Autodesk Inventor part; units mm, degrees
ref_plane "YZ Plane" through (0, 0, 0) normal (1, 0, 0) x (0, 1, 0)
ref_plane "XZ Plane" through (0, 0, 0) normal (0, 1, 0) x (-1, 0, 0)
ref_plane "XY Plane" through (0, 0, 0) normal (0, 0, 1) x (1, 0, 0)
sketch "Sketch1" plane through (0, 0, 0) normal (0, 0, 1) x (1, 0, 0)
  line L0 (-14, 8) -> (14, 8)
  line L1 (14, 8) -> (14, -8)
  line L2 (14, -8) -> (-14, -8)
  line L3 (-14, -8) -> (-14, 8)
  circle A0 centre (-9, 4) radius 1.6
  circle A1 centre (-9, -4) radius 1.6
  circle A2 centre (9, -4) radius 1.6
  circle A3 centre (9, 4) radius 1.6
  point P0 (0, 0)
  point P1 (0, 8)
  point P2 (-14, 0)
  dimension "d0" = 28
  dimension "d1" = 16
  dimension "d2" = 18
  dimension "d3" = 9
  dimension "d4" = 8
  dimension "d5" = 4
  dimension "d6" = 3.2
extrude "Extrusion1" add sketch "Sketch1" along normal blind 3
sketch "Sketch2" plane through (0, 0, 3) normal (0, 0, 1) x (1, 0, 0)
  line L0 (-4, -3.5) -> (-4, 3.5)
  line L1 (-4, 3.5) -> (-2, 8)
  line L2 (14, 8) -> (-14, 8)
  line L3 (-2, 8) -> (2, 8)
  line L4 (2, 8) -> (4, 3.5)
  line L5 (4, 3.5) -> (4, -3.5)
  line L6 (14, 8) -> (-14, 8)
  line L7 (4, -3.5) -> (2, -8)
  line L8 (-14, -8) -> (14, -8)
  line L9 (2, -8) -> (-2, -8)
  line L10 (-2, -8) -> (-4, -3.5)
  point P0 (0, 0)
  point P1 (-4, 0)
  point P2 (4, 0)
  point P3 (0, 8)
  dimension "d9" = 8
  dimension "d10" = 4
  dimension "d11" = 7
extrude "Extrusion2" add sketch "Sketch2" along normal blind 14
sketch "Sketch3" plane through (-4, -3.5, 3) normal (-1, 0, 0) x (0, 0, 1)
  circle A0 centre (11, 3.5) radius 2.05
  line L0 (14, 7) -> (14, 0)
  point P0 (-3, 3.5)
  point P1 (14, 3.5)
  dimension "d14" = 3
  dimension "d15" = 4.1
extrude "Extrusion3" cut sketch "Sketch3" against normal through all
sketch "Sketch4" plane through (0, 0, 17) normal (0, 0, 1) x (1, 0, 0)
  circle A0 centre (0, 0) radius 1.4
  dimension "d18" = 2.8
extrude "Extrusion4" cut sketch "Sketch4" against normal blind 3
properties part number "Guider"
Work out the finished part from the listing and answer in its coordinate system (mm). A direction names the side the tool comes from. Coordinates: 2 decimals unless noted, no trailing zeros. Order: outer loops, then holes, each group sorted by start corner. A loop starts at its lowest first (then second) coordinate and runs counter-clockwise, first axis right, second up. Notation, with made-up numbers: (50.5, 84.5) - (58.5, 84.5) arc R14 cw to (58.5, 92.5) - close; hole circle Ø4 at (35, -6). An arc over 180 degrees is marked (long way). Answer as a JSON object with one key per item and string values.
1. Find section C-C on y = 4. Determine the outline of the cut face in (x, z), plus the area to 3 significant figures.
Output values:
{"outline": "(-14, 0) - (-10.6, 0) - (-10.6, 3) - (-14, 3) - close; (-7.4, 0) - (7.4, 0) - (7.4, 3) - (3.78, 3) - (3.78, 17) - (-3.78, 17) - (-3.78, 3) - (-7.4, 3) - close; (10.6, 0) - (14, 0) - (14, 3) - (10.6, 3) - close", "area": "171 mm²"}
2. Consider line 1 (Y direction, x = -9, z = 0.6); line 2 (Y direction, x = 1.25, z = 14); line 3 (X direction, y = 0, z = 16.2). Determine where each line is inside the solid, lowest interval first.
Output values:
{"line 1": "y = -8 to -5.6, -2.4 to 2.4, 5.6 to 8", "line 2": "y = -8 to -2.05, 2.05 to 8", "line 3": "x = -4 to -1.4, 1.4 to 4"}
3. Each of these flat-tipped pins is pushed along its axis until it touches: P1, Ø6.5, axis at y = 0, z = 14, coming from the -X side; P2, Ø5, axis at x = -9, z = 6.5, coming from the +Y side; P3, Ø7.5, axis at y = -1, z = 12.5, coming from the +X side. Where does it stop, or does it pass through?
Output values:
{"P1": "stops at x = -4", "P2": "passes through", "P3": "stops at x = 4"}
4. Find section B-B on z = 14. Determine the outline of the cut face in (x, y).
Output values:
{"outline": "(-4, -3.5) - (-2, -8) - (2, -8) - (4, -3.5) - (4, -2.05) - (-4, -2.05) - close; (-4, 2.05) - (4, 2.05) - (4, 3.5) - (2, 8) - (-2, 8) - (-4, 3.5) - close"}
5. Find section D-D on z = 9. Determine the outline of the cut face in (x, y), plus the area to 3 significant figures.
Output values:
{"outline": "(-4, -3.5) - (-2, -8) - (2, -8) - (4, -3.5) - (4, 3.5) - (2, 8) - (-2, 8) - (-4, 3.5) - close", "area": "110 mm²"}
6. A tool of negligible diameter and unlimited length cuts with its end or side. For faces 1 (the face through (-2.986, -5.781, 9.902)), 2 (the face through (2.986, 5.781, 9.902)), 3 (the face through (-10.6, 3.93, 1.48)), 4 (the face through (-4, 0, 10)), from which of +Z, -Z, +X, -X, +Y, -Y can it reach the whole face along a straight path? Write none if from no direction.
Output values:
{"face 1": "+Z, -X, -Y", "face 2": "+Z, +X, +Y", "face 3": "+Z, -Z", "face 4": "+Z, -X, +Y, -Y"}
7. Find section A-A on x = -9. Determine the outline of the cut face in (y, z), plus the area to 3 significant figures.
Output values:
{"outline": "(-8, 0) - (-5.6, 0) - (-5.6, 3) - (-8, 3) - close; (-2.4, 0) - (2.4, 0) - (2.4, 3) - (-2.4, 3) - close; (5.6, 0) - (8, 0) - (8, 3) - (5.6, 3) - close", "area": "28.8 mm²"}
8. The mould has two halves that part along X. Classify faces 5 (the face through (7.4, -4.07, 1.48)), 6 (the face through (-1.4, 0.06, 16.43)), 7 (the face through (-2, 0, 17)), 8 (the face through (-3.014, 5.719, 9.902)): +X half, -X half, draft (parallel to the pull), parting line (faces both ways), or undercut.
Output values:
{"face 5": "undercut", "face 6": "undercut", "face 7": "draft", "face 8": "-X half"}
